Part model, mm, in its own coordinate system. A direction names the side the tool comes from. Round coordinates to 2 decimals unless told otherwise and drop trailing zeros. Order: outer loops, then holes, each group sorted by start corner. A loop starts at its lowest first (then second) coordinate and runs counter-clockwise, first axis right, second up. Notation, with made-up numbers: (-0.5, -37.75) - (43.5, -37.75) arc R34 cw to (43.5, -2.75) - close; hole circle Ø6 at (14.5, 69). An arc over 180 degrees is marked (long way). Answer as a JSON object with one key per item and string values.
Solid Edge part; units mm, degrees
sketch "Sketch1" plane through (0, 0, 0) normal (0, -1, 0) x (1, 0, 0)
  line L0 (0, 45) -> (30, 45)
  line L1 (30, 45) -> (30, 35)
  line L2 (30, 35) -> (37.5, 35)
  line L3 (37.5, 35) -> (37.5, 0)
  line L4 (0, 0) -> (37.5, 0)
revolve "RevolvedProtrusion1" add sketch "Sketch1" angle 360 about axis through (0, 0, 0) along (0, 0, 1)
chamfer "Chamfer_1" distance 1 angle 60 2 edges at (-37.5, 0, 35) (-30, 0, 45) measured on face at (25.75, -24.25, 35) measured on face at (20.6, -19.4, 45)
sketch "Sketch2" plane through (0, 0, 0) normal (0, 0, -1) x (0, 1, 0)
  line L0 (-21.5, -21.5) -> (21.5, -21.5)
  line L1 (21.5, -21.5) -> (21.5, 21.5)
  line L2 (21.5, 21.5) -> (-21.5, 21.5)
  line L3 (-21.5, 21.5) -> (-21.5, -21.5)
  dimension "D1" = 21.5
extrude "ExtrudedCutout_1" cut sketch "Sketch2" against normal blind 38
hole "Hole_1" at (0, 0, 45) direction (0, 0, -1) diameter 25 end up to next
hole "Hole_2" at (15.5, -15.5, 45) direction (0, 0, -1) diameter 3.6 end up to next counterbore diameter 6.5 counterbore depth 3.5
hole "Hole1" at (15.5, 15.5, 45) direction (0, 0, -1) diameter 3.6 end up to next counterbore diameter 6.5 counterbore depth 3.5
hole "Hole2" at (-15.5, 15.5, 45) direction (0, 0, -1) diameter 3.6 end up to next counterbore diameter 6.5 counterbore depth 3.5
hole "Hole3" at (-15.5, -15.5, 45) direction (0, 0, -1) diameter 3.6 end up to next counterbore diameter 6.5 counterbore depth 3.5
sketch "Sketch3" plane through (0, 0, 0) normal (0, 0, -1) x (-1, 0, 0)
  line L0 (0, 12.5) -> (0, -12.5)
  line L1 (0, -12.5) -> (-50, -12.5)
  line L2 (-50, -12.5) -> (-50, 12.5)
  line L3 (-50, 12.5) -> (0, 12.5)
  dimension "D1" = 50
  dimension "D2" = 50
extrude "ExtrudedCutout_2" cut sketch "Sketch3" against normal blind 15
sketch "Sketch4" plane through (-1.0723, 0, 0) normal (0, 0, -1) x (0, -1, 0)
  line L0 (-40, 23.9277) -> (-40, -26.0723)
  line L1 (-40, -26.0723) -> (-25, -29.0232)
  line L2 (-25, -29.0232) -> (-25, 26.8785)
  line L3 (-25, 26.8785) -> (-40, 23.9277)
  dimension "D1" = 40
extrude "ExtrudedProtrusion_1" add sketch "Sketch4" against normal blind 20
hole "Hole_6" at (-15, 40, 10) direction (0, -1, 0) diameter 4.8 end up to next
hole "Hole4" at (15, 40, 10) direction (0, -1, 0) diameter 4.8 end up to next
mirror "Mirror1" about plane through (0, 0, 0) normal (0, -1, 0) of "ExtrudedProtrusion_1", "Hole_6", "Hole4"
properties material "Polyethylene, low density"
Item 1: Cut at A-A (y = 0). Write the cut outline in (x, z).
Taken from the geometry:
{"outline": "(-37.5, 0) - (-21.5, 0) - (-21.5, 38) - (-12.5, 38) - (-12.5, 45) - (-29, 45) - (-30, 43.27) - (-30, 35) - (-36.5, 35) - (-37.5, 33.27) - close; (12.5, 38) - (21.5, 38) - (21.5, 15) - (37.5, 15) - (37.5, 33.27) - (36.5, 35) - (30, 35) - (30, 43.27) - (29, 45) - (12.5, 45) - close"}
Item 2: Two-plate mould, pull along X, no slides. Class faces 6 (the flat face through (0, -38, 20)), 7 (the flat face through (-26.496, 32.395, 9.86)), 8 (the cylindrical face through (17.285, 15.734, 39.774)): pulls with the +X half, pulls with the -X half, needs draft (parallel to the pull), parting line crosses it, or undercut.
Taken from the geometry:
{"face 6": "needs draft", "face 7": "pulls with the -X half", "face 8": "undercut"}
Item 3: Drop flat-ended pins along their axis: P1, Ø3, axis at x = -1.5, z = 39, coming from the +Y side; P2, Ø8.5, axis at x = 15.5, y = -15.5, coming from the -Z side; P3, Ø10, axis at x = -29.5, z = 36, coming from the +Y side. Give the stop position or say it passes through.
Taken from the geometry:
{"P1": "y = 30", "P2": "z = 38", "P3": "y = 27.67"}
Item 4: Tool access for faces 1 (the flat face through (-21.5, 0, 19)), 2 (the flat face through (0, 38, 20)), 3 (the flat face through (12, -6, 45)), 4 (the cylindrical face through (-18.722, 15.923, 43.226)), 5 (the flat face through (-26, 1, 0)): list every direction of +Z, -Z, +X, -X, +Y, -Y with a clear straight run to the whole face (end or side of a thin tool).
Taken from the geometry:
{"face 1": "-Z", "face 2": "+Z, +Y", "face 3": "+Z, +X, -X, +Y, -Y", "face 4": "+Z", "face 5": "-Z, +X, -X, +Y, -Y"}
Item 5: Probe L1, parallel to Z at x = -15, y = -33; L2, parallel to Y at x = -15.5, z = 43.1; L3, parallel to Y at x = 17, z = 6. List the from-to ranges inside material, lowest first. Write a range as from..to.
Taken from the geometry:
{"L1": "0..7.6, 12.4..35", "L2": "-25.69..-18.75, -12.25..12.25, 18.75..25.69", "L3": "-40..-21.5, 21.5..40"}
Item 6: Cut at D-D (y = 31). State how many separate pieces and enclosed holes the cut face has, plus the area to 3 significant figures.
Taken from the geometry:
{"separate pieces": "1", "enclosed holes": "2", "area": "1,660 mm2"}
Item 7: Cut at B-B (z = 24). Write the cut outline in (x, y).
Taken from the geometry:
{"outline": "circle Ø75 at (0, 0); hole (-21.5, -21.5) - (21.5, -21.5) - (21.5, 21.5) - (-21.5, 21.5) - close"}
